Geometry check sheet. Reference: the model listing, model coordinates, mm. Round coordinates to 2 decimals unless told otherwise and drop trailing zeros. Order: outer loops, then holes, each group sorted by start corner. A loop starts at its lowest first (then second) coordinate and runs counter-clockwise, first axis right, second up. Notation, with made-up numbers: (21.25, 9) - (26.25, 9) arc R10 ccw to (26.25, 16) - close; hole circle Ø6 at (69, 3.5). An arc over 180 degrees is marked (long way). Use a Markdown table: item, result. Add a question column.
(1) Thickness scan on line 1 along X through (y, z) = (-88, 6.35); line 2 along X through (y, z) = (75, 5); line 3 along Y through (x, z) = (67.5, 7.5). Record the ranges inside material, lowest first. Write a range as [from, to].
(2) Section check A-A on x = 7. Record the boundary of the cut face in (y, z).
(3) Gauge pin test, flat ends, axial feed: P1, Ø5, axis at x = -53.5, z = 6.35, coming from the +Y side; P2, Ø1.5, axis at x = -27.5, z = 8.5, coming from the +Y side; P3, Ø6.5, axis at x = 67.5, z = 9.5, coming from the +Y side; P4, Ø1.9, axis at x = 69.5, y = -72.5, coming from the -Z side. Record the tip position at first contact, or that the pin passes through.
(4) Section check B-B on y = 50. Record the boundary of the cut face in (x, z).
```python
from build123d import *

# Parameters (mm, degrees)
EXTRUDE1_DEPTH = 12.7
SKETCH3_R      = 3.175
EXTRUDE2_DEPTH = 12.7
SKETCH4_R      = 3.175
EXTRUDE3_DEPTH = 6.35
SKETCH6_W      = 19.05
SKETCH6_H      = 0.635
EXTRUDE4_DEPTH = 6.35


with BuildPart() as part:
    # Sketch1 → Extrude1 (new body)
    with BuildSketch(Plane.XY):
        Polygon((-61.751637834, 93.380203425), (-61.751637834, -93.380203425), (61.751637834, -93.380203425), (80.801637834, -93.380203425), (80.801637834, -67.980203425), (61.751637834, -67.980203425), align=None)
    extrude(amount=EXTRUDE1_DEPTH)

    # Sketch3 → Extrude2 (cut)
    with BuildSketch(Plane.XZ.offset(93.380203425)):
        with Locations(Location((-53.500521912, 6.35, 0), (0, 0, 270))):
            Circle(SKETCH3_R)
        with Locations(Location((48.099478088, 6.35, 0), (0, 0, 270))):
            Circle(SKETCH3_R)
    extrude(amount=-EXTRUDE2_DEPTH, mode=Mode.SUBTRACT)

    # Sketch4 → Extrude3 (cut)
    with BuildSketch(Plane(origin=(6.12959486, 4.691516702, 0), x_dir=(0, 0, -1), z_dir=(0.7940964904073088, 0.6077917109691402, 0))):
        with Locations(Location((-6.128651302, 95.810025428, 0), (0, 0, 90))):
            Circle(SKETCH4_R)
        with Locations(Location((-6.128651302, 10.085025428, 0), (0, 0, 90))):
            Circle(SKETCH4_R)
    extrude(amount=-EXTRUDE3_DEPTH, mode=Mode.SUBTRACT)

    # Sketch6 → Extrude4 (cut)
    with BuildSketch(Plane(origin=(0, -67.980203425, 0), x_dir=(1, 0, 0), z_dir=(0, 1, 0))):
        with Locations((71.276637834, -6.6675)):
            Rectangle(SKETCH6_W, SKETCH6_H)
    extrude(amount=-EXTRUDE4_DEPTH, mode=Mode.SUBTRACT)


solid = part.part
```
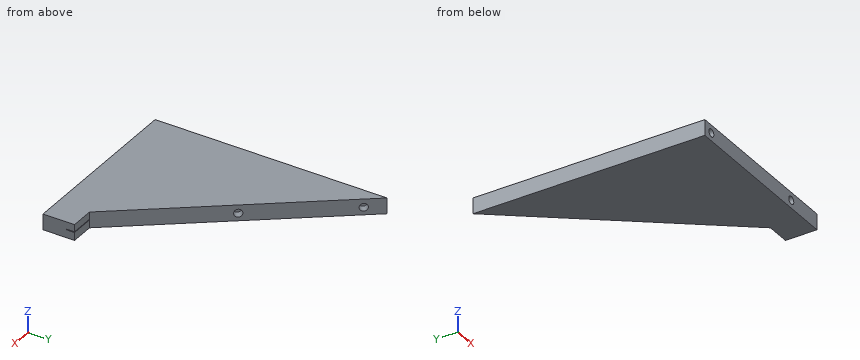
Check sheet entries:
| question | item | result |
|---|---|---|
| 1 | line 1 | x = [-61.75, -56.68], [-50.33, 44.92], [51.27, 80.8] |
| 1 | line 2 | x = [-61.75, -55.68], [-54.76, -47.68] |
| 1 | line 3 | y = [-93.38, -67.98] |
| 2 | outline | (-93.38, 0) - (3.55, 0) - (3.55, 12.7) - (-93.38, 12.7) - close |
| 3 | P1 | stops at y = 85.87 |
| 3 | P2 | stops at y = 49.61 |
| 3 | P3 | stops at y = -67.98 |
| 3 | P4 | stops at z = 0 |
| 4 | outline | (-61.75, 0) - (-28.55, 0) - (-28.55, 12.7) - (-61.75, 12.7) - close |
